For this review, take the finished solid that the model builds, in its own axes (mm). Face numbers are marked on the shaded views. A direction names the side the tool comes from. Round coordinates to 2 decimals unless told otherwise and drop trailing zeros. Order: outer loops, then holes, each group sorted by start corner. A loop starts at its lowest first (then second) coordinate and runs counter-clockwise, first axis right, second up.
from build123d import *

# Parameters (mm, degrees)
CHAMFER1_SIZE      = 0.2
CUT_EXTRUDE1_START = 0.5
CUT_EXTRUDE1_DEPTH = 10
FILLET1_R          = 0.2


with BuildPart() as part:
    # Sketch1 → Revolve1 (revolve)
    with BuildSketch(Plane.XY, mode=Mode.PRIVATE) as revolve1_sk:
        with BuildLine():
            Line((1.25, 0), (2.25, 0))
            Line((2.25, 0), (2.25, 0.3))
            ThreePointArc((2.25, 0.3), (1.73223122, 1.011699188), (1, 1.5))
            Line((1, 1.5), (0, 1.5))
            Line((0, 1.5), (0, -8))
            Line((0, -8), (1.25, -8))
            Line((1.25, -8), (1.25, 0))
        make_face()
    revolve(revolve1_sk.sketch.rotate(Axis((0, 21.344098617, 0), (0, -1, 0)), 90), axis=Axis((0, 21.344098617, 0), (0, -1, 0)))

    # Chamfer1
    chamfer1_edges = [part.edges().sort_by_distance(p)[0] for p in [
        (0, -8, -1.25),
    ]]
    chamfer(chamfer1_edges, length=CHAMFER1_SIZE)

    # Sketch2 → Cut-Extrude1 (cut)
    with BuildSketch(Plane(origin=(0, 0, 0), x_dir=(1, 0, 0), z_dir=(0, 1, 0)).offset(CUT_EXTRUDE1_START)):
        Polygon((0.433012702, -0.75), (0.866025404, 0), (0.433012702, 0.75), (-0.433012702, 0.75), (-0.866025404, 0), (-0.433012702, -0.75), align=None)
    extrude(amount=CUT_EXTRUDE1_DEPTH, mode=Mode.SUBTRACT)

    # Fillet1
    fillet1_edges = [part.edges().sort_by_distance(p)[0] for p in [
        (0, 0, -1.25),
    ]]
    fillet(fillet1_edges, radius=FILLET1_R)


solid = part.part
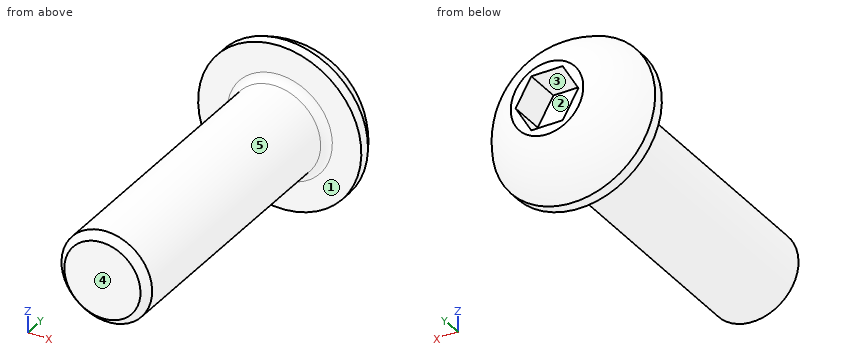
(1) Add section B-B on y = 0.75. Give the boundary of the cut face in (x, z), plus the area to 3 significant figures.
(2) Draft analysis for pull direction Z (two halves, no side actions). For the marked faces 3, 4 and 5, state which applies: pulls with the +Z half, pulls with the -Z half, needs draft (parallel to the pull), parting line crosses it, or undercut.
(3) Clearance check with flat-ended pins moving along their axes: P1, Ø2, axis at x = 0.5, z = 2, coming from the +Y side; P2, Ø2, axis at y = -5.5, z = 0, coming from the +X side; P3, Ø1, axis at y = -6.5, z = -1.5, coming from the -X side. State where each tip first meets the part, or that it passes through.
(4) Wall thickness on L1, parallel to X at y = 0.25, z = 0.1; L2, parallel to Z at x = 1, y = -0.5; L3, parallel to Z at x = 0.5, y = -4.5: over which ranges is each line inside the solid? List them lowest first.
(5) Add section D-D on y = -3.5. Give the boundary of the cut face in (x, z), plus the area to 3 significant figures.
(6) Add section C-C on z = -2. Give the boundary of the cut face in (x, y).
(7) Add section A-A on x = 0. Give the boundary of the cut face in (y, z), plus the area to 3 significant figures.
(8) Tool access review of the marked faces 1 and 2: name each direction out of +Z, -Z, +X, -X, +Y, -Y from which nothing blocks a thin tool from reaching the whole face with its end or side.
Here are the results:
1. outline: circle Ø3.94 at (0, 0); hole (-0.87, 0) - (-0.43, -0.75) - (0.43, -0.75) - (0.87, 0) - (0.43, 0.75) - (-0.43, 0.75) - close
1. area: 10.2 mm2
2. face 3: undercut
2. face 4: needs draft
2. face 5: parting line crosses it
3. P1: stops at y = 1.47
3. P2: stops at x = 1.25
3. P3: stops at x = -0.75
4. L1: x = -2.25 to 2.25
4. L2: z = -0.75 to 0.75
4. L3: z = -1.15 to 1.15
5. outline: circle Ø2.5 at (0, 0)
5. area: 4.91 mm2
6. outline: (-1.03, 0) - (1.03, 0) - (1.03, 0.3) arc R1.5 ccw to (-1.03, 0.3) - close
7. outline: (-8, -1.05) - (-7.8, -1.25) - (-0.2, -1.25) arc R0.2 cw to (0, -1.45) - (0, -2.25) - (0.3, -2.25) arc R2.5 ccw to (1.5, -1) - (1.5, -0.75) - (0.5, -0.75) - (0.5, 0.75) - (1.5, 0.75) - (1.5, 1) arc R2.5 ccw to (0.3, 2.25) - (0, 2.25) - (0, 1.45) arc R0.2 cw to (-0.2, 1.25) - (-7.8, 1.25) - (-8, 1.05) - close
7. area: 24.1 mm2
8. face 1: -Y
8. face 2: +Y
